Read the model definition and answer for the solid it produces. Units are mm, in the model's axes. A direction names the side the tool comes from. Round coordinates to 2 decimals unless told otherwise and drop trailing zeros. Loops run counter-clockwise (first coordinate to the right, second up) from the corner with the lowest first, then second, coordinate; pieces in that order, holes last. Notation, with made-up numbers: M -8.75,85.5 L 4.25,85.5 A19 cw 4.25,103.5 Z; hole C 54.25,45 d8. An arc over 180 degrees is marked long. Answer as CSV lines item,"result".
```python
from build123d import *

# Parameters (mm, degrees)
F0_R          = 2
F1_DEPTH      = 6
F2_W          = 7.8
F2_H          = 78
F3_DEPTH      = 12
F4_R          = 2
F5_DEPTH      = 12
F6_W          = 2.5
F6_H          = 7
F7_DEPTH      = 33.901
F8_R          = 1.5
F9_DEPTH      = 39.001
F9_DEPTH_BACK = 39.001
F10_DEPTH     = 2.5
F11_SIZE      = 1
F12_R         = 1
F13_SIZE      = 1
F14_SIZE      = 1
F15_W         = 13.75
F15_H         = 4
F16_DEPTH     = 2


# Not quite as in the source:
# - a feature names something its author has since deleted; it is built from what else it names


with BuildPart() as f1:
    # F0 (on Front) → F1 (new body)
    with BuildSketch(Plane.XZ):
        with BuildLine():
            Line((22.3473393815, 1.2260917259), (13.7473393815, 35.2260917259))
            ThreePointArc((13.7473393815, 35.2260917259), (11.9716071828, 37.9452793709), (8.9, 39))
            Line((8.9, 39), (-8.9, 39))
            ThreePointArc((-8.9, 39), (-11.1047505583, 38.4876580725), (-12.8576666563, 37.0556299903))
            Line((-12.8576666563, 37.0556299903), (-29.4788333281, 15.5278149952))
            ThreePointArc((-29.4788333281, 15.5278149952), (-29.8661237626, 14.8071296921), (-30, 14))
            Line((-30, 14), (-30, 0))
            ThreePointArc((-30, 0), (-29.8782578321, -1.0966314436), (-29.5189597908, -2.1398603715))
            Line((-29.5189597908, -2.1398603715), (-13.4189597908, -36.1398603715))
            ThreePointArc((-13.4189597908, -36.1398603715), (-11.5740136632, -38.2248847237), (-8.9, -39))
            Line((-8.9, -39), (8.9, -39))
            ThreePointArc((8.9, -39), (11.9716071828, -37.9452793709), (13.7473393815, -35.2260917259))
            Line((13.7473393815, -35.2260917259), (22.3473393815, -1.2260917259))
            ThreePointArc((22.3473393815, -1.2260917259), (22.5, 0), (22.3473393815, 1.2260917259))
        make_face()
        with Locations((-8.9, -34)):
            Circle(F0_R, mode=Mode.SUBTRACT)
        with Locations((-8.9, -10.1)):
            Circle(F0_R, mode=Mode.SUBTRACT)
        with Locations((8.9, -34)):
            Circle(F0_R, mode=Mode.SUBTRACT)
        with Locations((8.9, -10.1)):
            Circle(F0_R, mode=Mode.SUBTRACT)
        with Locations((-25, 0)):
            Circle(F0_R, mode=Mode.SUBTRACT)
        with BuildLine():
            ThreePointArc((-20.5, 9.25), (-19.25, 8), (-20.5, 6.75))
            Line((-20.5, 6.75), (-27.5, 6.75))
            ThreePointArc((-27.5, 6.75), (-28.75, 8), (-27.5, 9.25))
            Line((-27.5, 9.25), (-20.5, 9.25))
        make_face(mode=Mode.SUBTRACT)
        with BuildLine():
            ThreePointArc((-27.5, 12.75), (-28.75, 14), (-27.5, 15.25))
            Line((-27.5, 15.25), (-20.5, 15.25))
            ThreePointArc((-20.5, 15.25), (-19.25, 14), (-20.5, 12.75))
            Line((-20.5, 12.75), (-27.5, 12.75))
        make_face(mode=Mode.SUBTRACT)
        with Locations((-8.9, 10.1)):
            Circle(F0_R, mode=Mode.SUBTRACT)
        with Locations((-8.9, 34)):
            Circle(F0_R, mode=Mode.SUBTRACT)
        with Locations((8.9, 10.1)):
            Circle(F0_R, mode=Mode.SUBTRACT)
        with Locations((17.5, 0)):
            Circle(F0_R, mode=Mode.SUBTRACT)
        with Locations((8.9, 34)):
            Circle(F0_R, mode=Mode.SUBTRACT)
    extrude(amount=F1_DEPTH)

    # F2 (on face) → F3 (join)
    with BuildSketch(Plane.XZ.offset(6)):
        Rectangle(F2_W, F2_H)
    extrude(amount=F3_DEPTH)

    # F4 (on face) → F5 (cut, through all)
    with BuildSketch(Plane.XZ.offset(18)):
        Circle(F4_R)
    extrude(amount=-F5_DEPTH, mode=Mode.SUBTRACT)

    # F6 (on face) → F7 (cut, through all)
    with BuildSketch(Plane.YZ.offset(3.9)):
        with Locations((-13.75, 0)):
            Rectangle(F6_W, F6_H)
    extrude(amount=-F7_DEPTH, mode=Mode.SUBTRACT)

    # F8 (on Top) → F9 (cut, two sides)
    with BuildSketch(Plane.XY) as f9_sk:
        with Locations((0, -10)):
            Circle(F8_R)
    extrude(amount=-F9_DEPTH, mode=Mode.SUBTRACT)
    extrude(f9_sk.sketch, amount=F9_DEPTH_BACK, mode=Mode.SUBTRACT)

    # F10 (add): a face of the model
    f10_faces = [f1.faces().sort_by_distance(p)[0] for p in [
        (0, -6, 0),
    ]]
    extrude(f10_faces, amount=F10_DEPTH)

    # F11
    f11_edges = [f1.edges().sort_by_distance(p)[0] for p in [
        (3.9, -18, 0),
        (-3.9, -18, 0),
    ]]
    chamfer(f11_edges, length=F11_SIZE)

    # F12
    f12_edges = [f1.edges().sort_by_distance(p)[0] for p in [
        (-3.9, -6, 0),
        (3.9, -6, 0),
    ]]
    fillet(f12_edges, radius=F12_R)

    # F13 (call 1 of 4: OpenCascade refuses the feature's edges together)
    f13_edges = [f1.edges().sort_by_distance(p)[0] for p in [
        (18.047339, -6, 18.226092),
    ]]
    chamfer(f13_edges, length=F13_SIZE)

    # F13#2 (call 2 of 4)
    f13_2_edges = [f1.edges().sort_by_distance(p)[0] for p in [
        (0, -18, -39),
    ]]
    chamfer(f13_2_edges, length=F13_SIZE)

    # F13#3 (call 3 of 4)
    f13_3_edges = [f1.edges().sort_by_distance(p)[0] for p in [
        (0, -18, 39),
    ]]
    chamfer(f13_3_edges, length=F13_SIZE)

    # F13#4 (call 4 of 4)
    f13_4_edges = [f1.edges().sort_by_distance(p)[0] for p in [
        (-30, -6, 7),
    ]]
    chamfer(f13_4_edges, length=F13_SIZE)

    # F14
    f14_edges = [f1.edges().sort_by_distance(p)[0] for p in [
        (-1.5, -10, 39),
    ]]
    chamfer(f14_edges, length=F14_SIZE)

    # F15 (on face) → F16 (cut)
    with BuildSketch(Plane(origin=(0, 0, 0), x_dir=(-1, 0, 0), z_dir=(0, 1, 0))):
        with BuildLine():
            Line((29.1142693598, 16), (16.25, 16))
            Line((16.25, 16), (16.25, 12))
            Line((16.25, 12), (30, 12))
            Line((30, 12), (30, 14))
            ThreePointArc((30, 14), (29.8661237626, 14.8071296921), (29.4788333281, 15.5278149952))
            Line((29.4788333281, 15.5278149952), (29.1142693598, 16))
        make_face()
        with BuildLine():
            Line((20.5, 15.25), (27.5, 15.25))
            ThreePointArc((27.5, 15.25), (28.75, 14), (27.5, 12.75))
            Line((27.5, 12.75), (20.5, 12.75))
            ThreePointArc((20.5, 12.75), (19.25, 14), (20.5, 15.25))
        make_face(mode=Mode.SUBTRACT)
        with Locations((23.125, 8)):
            Rectangle(F15_W, F15_H)
        with BuildLine():
            Line((27.5, 6.75), (20.5, 6.75))
            ThreePointArc((20.5, 6.75), (19.25, 8), (20.5, 9.25))
            Line((20.5, 9.25), (27.5, 9.25))
            ThreePointArc((27.5, 9.25), (28.75, 8), (27.5, 6.75))
        make_face(mode=Mode.SUBTRACT)
    extrude(amount=-F16_DEPTH, mode=Mode.SUBTRACT)


solid = f1.part
```
1) Straight lines are drawn through the part: line 1 (Z direction, x = 8.9, y = -4); line 2 (Y direction, x = -13, z = 19); line 3 (X direction, y = -16.5, z = -13). For each, find the intervals that lie inside material, in ascending order.
Evaluation:
line 1,"z = -39 to -36, -32 to -12.1, -8.1 to 8.1, 12.1 to 32, 36 to 39"
line 2,"y = -6 to 0"
line 3,"x = -3.9 to 3.9"
2) A tool of negligible diameter and unlimited length cuts with its end or side. For faces 5 (the flat face through (-23, -1, 6)), 6 (the flat face through (-14, -6, 1)), 7 (the cylindrical face through (-19.25, -3.97, 8.03)), 8 (the cylindrical face through (-2, -11, 0)), 9 (the cylindrical face through (-11.08, -2.46, 38.5)), from which of +Z, -Z, +X, -X, +Y, -Y can it reach the whole face along a straight path? Write none if from no direction.
Evaluation:
face 5,"-X, +Y"
face 6,"+Z, -Z, -X, -Y"
face 7,"+Y, -Y"
face 8,"-Y"
face 9,"+Z, -X, +Y, -Y"
3) Find section A-A, the plane z = 17. Give the vertices of the cut face in (x, y), then the cut area to 3 significant figures.
Evaluation:
outline,"M -28.34,-5 L -27.08,-6 L -4.9,-6 A1 cw -3.9,-7 L -3.9,-17 L -2.9,-18 L 2.9,-18 L 3.9,-17 L 3.9,-7 A1 cw 4.9,-6 L 17.33,-6 L 18.36,-5 L 18.36,0 L -28.34,0 Z; hole C 0,-10 d3"
area,"365 mm^2"
4) Determine the mould class of faces 1 (the cylindrical face through (-0.325, -11.464, 19.405)), 2 (the cylindrical face through (-9.334, -2.958, 32.048)), 3 (the conical face through (-3.92, -6, -38.4)), 4 (the flat face through (17.63, -5.49, 17.87)) for opening direction Z: released by +Z, released by -Z, zero draft, split by the parting line, or undercut.
Evaluation:
face 1,"zero draft"
face 2,"undercut"
face 3,"released by -Z"
face 4,"released by +Z"
5) Find section B-B, the plane z = -7. Give the vertices of the cut face in (x, y), then the cut area to 3 significant figures.
Evaluation:
outline,"M -27.22,-5 L -26.11,-6 L -4.9,-6 A1 cw -3.9,-7 L -3.9,-17 L -2.9,-18 L 2.9,-18 L 3.9,-17 L 3.9,-7 A1 cw 4.9,-6 L 19.86,-6 L 20.89,-5 L 20.89,0 L -27.22,0 Z; hole C 0,-10 d3"
area,"374 mm^2"
6) Each of these flat-tipped pins is pushed along its axis until it touches: P1, Ø2, axis at x = -24, y = -0.5, coming from the +Z side; P2, Ø6, axis at y = -8, z = -20, coming from the +X side; P3, Ø6, axis at x = 7, y = -11.5, coming from the +Z side; P4, Ø3, axis at y = -6, z = -27.5, coming from the -X side. Where does it stop, or does it pass through?
Evaluation:
P1,"stops at z = 23.92"
P2,"stops at x = 17.69"
P3,"passes through"
P4,"stops at x = -18.04"
